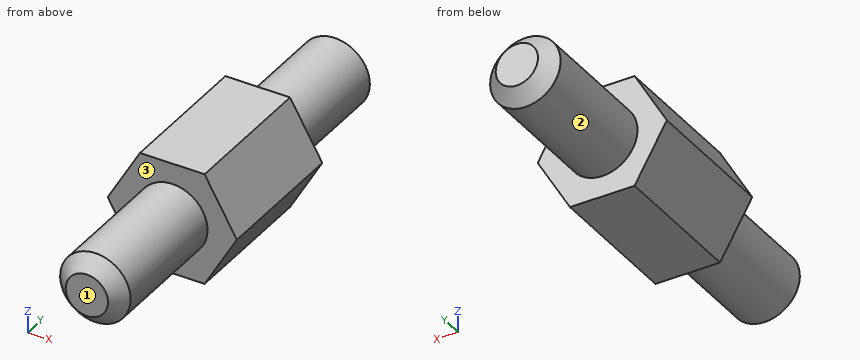
from build123d import *

# Parameters (mm, degrees)
EXTRUDE_1_DEPTH = 6
SKETCH_3_R      = 1.5
EXTRUDE_2_DEPTH = 6
EXTRUDE_START   = 6
SKETCH_4_R      = 1.5
EXTRUDE_3_DEPTH = 6
CHAMFER_1_SIZE  = 0.6


with BuildPart() as part:
    # Эскиз1 → Бобышка-Вытянуть1 (new body)
    with BuildSketch(Plane(origin=(0, 0, 0), x_dir=(1, 0, 0), z_dir=(0, 1, 0))):
        Polygon((-2.75, 0), (-1.375, 2.38156986), (1.375, 2.38156986), (2.75, 0), (1.375, -2.38156986), (-1.375, -2.38156986), align=None)
    extrude(amount=EXTRUDE_1_DEPTH)

    # Эскиз3 → Бобышка-Вытянуть2 (add)
    with BuildSketch(Plane(origin=(0, 6, 0), x_dir=(1, 0, 0), z_dir=(0, 1, 0))):
        with Locations(Location((0, 0, 0), (0, 0, 90))):
            Circle(SKETCH_3_R)
    extrude(amount=EXTRUDE_2_DEPTH)

    # Эскиз4 → Бобышка-Вытянуть3 (add)
    with BuildSketch(Plane.XZ.offset(EXTRUDE_START)):
        with Locations(Location((0, 0, 0), (0, 0, 270))):
            Circle(SKETCH_4_R)
    extrude(amount=-EXTRUDE_3_DEPTH)

    # Фаска1
    chamfer_1_edges = [part.edges().sort_by_distance(p)[0] for p in [
        (0, 12, 1.5),
        (0, -6, 1.5),
    ]]
    chamfer(chamfer_1_edges, length=CHAMFER_1_SIZE)


solid = part.part
Could you check a few things on this model? Use its own coordinates, in mm. Face numbers are marked on the shaded views. A direction names the side the tool comes from. Give positions to 0.01 mm unless a question says otherwise; leave off trailing zeros. Loops run counter-clockwise (first coordinate to the right, second up) from the corner with the lowest first, then second, coordinate; pieces in that order, holes last. Notation, with made-up numbers: (14, 87.25) -> (24, 87.25) arc R25 cw to (24, 109.25) -> close; hole circle Ø1 at (86, -8). An arc over 180 degrees is marked (long way). Return JSON: item names as keys, results as strings.
Item 1: I'm going to push flat-ended pins straight in: pin 1 (1.5 mm diameter, centred on x = -0.5, y = 9, fed in from +Z); pin 2 (3 mm diameter, centred on x = -1.5, y = -2, fed in from -Z). Where does each tip first touch, or does it pass through?
Geometry results:
{"pin 1": "stops at z = 1.5", "pin 2": "stops at z = -1.5"}
Item 2: If we section it at A-A on x = 0: List the corners of the cut face in (y, z) for me.
Geometry results:
{"outline": "(-6, -0.9) -> (-5.4, -1.5) -> (0, -1.5) -> (0, -2.38) -> (6, -2.38) -> (6, -1.5) -> (11.4, -1.5) -> (12, -0.9) -> (12, 0.9) -> (11.4, 1.5) -> (6, 1.5) -> (6, 2.38) -> (0, 2.38) -> (0, 1.5) -> (-5.4, 1.5) -> (-6, 0.9) -> close"}
Item 3: I need wall thicknesses on L1, parallel to Y at x = -2.05, z = -0.9; L2, parallel to X at y = -4.25, z = 0.6; L3, parallel to Z at x = -0.1, y = -0.5. Which ranges of each line are inside material? Lowest first, please. Write a range as from..to.
Geometry results:
{"L1": "y = 0..6", "L2": "x = -1.37..1.37", "L3": "z = -1.5..1.5"}
Item 4: If we section it at D-D on x = 1.9: List the corners of the cut face in (y, z) for me, plus the area to 3 significant figures.
Geometry results:
{"outline": "(0, -1.47) -> (6, -1.47) -> (6, 1.47) -> (0, 1.47) -> close", "area": "17.7 mm²"}
Item 5: Which directions (+Z, -Z, +X, -X, +Y, -Y) give clear straight access to the entire face, cutting with the end or side of a thin tool? Please do the marked faces 1, 2 and 3.
Geometry results:
{"face 1": "+Z, -Z, +X, -X, -Y", "face 2": "+Y", "face 3": "-Y"}
Item 6: If we section it at C-C on z = 1.95: List the corners of the cut face in (x, y) for me, plus the area to 3 significant figures.
Geometry results:
{"outline": "(-1.62, 0) -> (1.62, 0) -> (1.62, 6) -> (-1.62, 6) -> close", "area": "19.5 mm²"}
Item 7: If we section it at B-B on y = -2.75: List the corners of the cut face in (x, z) for me.
Geometry results:
{"outline": "circle Ø3 at (0, 0)"}
